Geometry check sheet. Reference: the model listing, model coordinates, mm. A direction names the side the tool comes from. Coordinates: 2 decimals unless noted, no trailing zeros. Write each loop counter-clockwise with the first axis right and the second up, starting at its lowest first coordinate (ties: lowest second). Pieces come first, ordered by that corner, then holes. Notation, with made-up numbers: (-37, 51.25) -> (-18, 51.25) arc R16 ccw to (-18, 55.25) -> close; hole circle Ø8 at (44.25, 0.25). An arc over 180 degrees is marked (long way). Answer in a Markdown table with one row per item. Add a question column.
Q1. Section check B-B, the plane y = -2.9. Count the separate pieces of the cut face and the enclosed holes in it, and give its area (3 significant figures).
Q2. Section check C-C, the plane x = 20. Record the boundary of the cut face in (y, z).
Q3. Gauge pin test, flat ends, axial feed: P1, Ø4, axis at x = 140, z = 12, coming from the +Y side; P2, Ø3, axis at x = 183.5, y = -4, coming from the +Z side; P3, Ø3, axis at y = -2, z = 84.5, coming from the -X side. Record the tip position at first contact, or that the pin passes through.
Q4. Section check A-A, the plane x = 70. Record the boundary of the cut face in (y, z), and give its area (3 significant figures).
Q5. Release check for a two-part mould opening along X. For faces 4 (the face through (60, -3, 20)), 5 (the face through (105, -3, 165)), 6 (the face through (135, -3, 104)), 7 (the face through (184, -3, 24)) record: pulls with the +X half, pulls with the -X half, needs draft (parallel to the pull), parting line crosses it, or undercut.
Q6. Section check D-D, the plane z = 80. Record the boundary of the cut face in (x, y).
Q7. Thickness scan on line 1 (Z direction, x = 190, y = -1.9); line 2 (Z direction, x = 140, y = -4.75); line 3 (Z direction, x = 68, y = -0.4). Record the ranges inside material, lowest first.
Q8. Tool access check on faces 1 (the face through (210, -3, 22)), 2 (the face through (38, -3, 45)), 3 (the face through (173, -3, 45)). Record the directions out of +Z, -Z, +X, -X, +Y, -Y that give a thin tool (end or side, any length) a straight path to the whole face; none if there is none.
```python
from build123d import *

# Parameters (mm, degrees)
SKETCH_R   = 10
SKETCH_R_2 = 5
SKETCH_R_3 = 6
SKETCH_R_4 = 1.75
PAD_DEPTH  = 6


with BuildPart() as part:
    # Sketch → Pad (new body)
    with BuildSketch(Plane.XZ):
        Polygon((0, 0), (210, 0), (210, 45), (135, 45), (135, 165), (75, 165), (75, 45), (0, 45), align=None)
        with Locations((70, 20)):
            Circle(SKETCH_R, mode=Mode.SUBTRACT)
        with Locations((140, 20)):
            Circle(SKETCH_R_2, mode=Mode.SUBTRACT)
        with Locations((20, 24)):
            Circle(SKETCH_R_3, mode=Mode.SUBTRACT)
        with Locations((190, 24)):
            Circle(SKETCH_R_3, mode=Mode.SUBTRACT)
        with Locations((140, 28)):
            Circle(SKETCH_R_4, mode=Mode.SUBTRACT)
        with Locations((132, 20)):
            Circle(SKETCH_R_4, mode=Mode.SUBTRACT)
        with Locations((140, 12)):
            Circle(SKETCH_R_4, mode=Mode.SUBTRACT)
        with Locations((148, 20)):
            Circle(SKETCH_R_4, mode=Mode.SUBTRACT)
    extrude(amount=PAD_DEPTH)


solid = part.part
```
Calculated:
| question | item | result |
|---|---|---|
| 1 | separate pieces | 1 |
| 1 | enclosed holes | 8 |
| 1 | area | 16,000 mm² |
| 2 | outline | (-6, 0) -> (0, 0) -> (0, 18) -> (-6, 18) -> close; (-6, 30) -> (0, 30) -> (0, 45) -> (-6, 45) -> close |
| 3 | P1 | stops at y = 0 |
| 3 | P2 | stops at z = 45 |
| 3 | P3 | stops at x = 75 |
| 4 | outline | (-6, 0) -> (0, 0) -> (0, 10) -> (-6, 10) -> close; (-6, 30) -> (0, 30) -> (0, 45) -> (-6, 45) -> close |
| 4 | area | 150 mm² |
| 5 | face 4 | undercut |
| 5 | face 5 | needs draft |
| 5 | face 6 | pulls with the +X half |
| 5 | face 7 | undercut |
| 6 | outline | (75, -6) -> (135, -6) -> (135, 0) -> (75, 0) -> close |
| 7 | line 1 | z = 0 to 18, 30 to 45 |
| 7 | line 2 | z = 0 to 10.25, 13.75 to 15, 25 to 26.25, 29.75 to 45 |
| 7 | line 3 | z = 0 to 10.2, 29.8 to 45 |
| 8 | face 1 | +Z, -Z, +X, +Y, -Y |
| 8 | face 2 | +Z, -X, +Y, -Y |
| 8 | face 3 | +Z, +X, +Y, -Y |
